Design review of the part shown in the three views and the two pictorial views. Dimensions are in mm from the part's minimum x, y and z. Give positions to 0.01 mm unless a question says otherwise; leave off trailing zeros. Write each loop counter-clockwise with the first axis right and the second up, starting at its lowest first coordinate (ties: lowest second). Pieces come first, ordered by that corner, then holes.
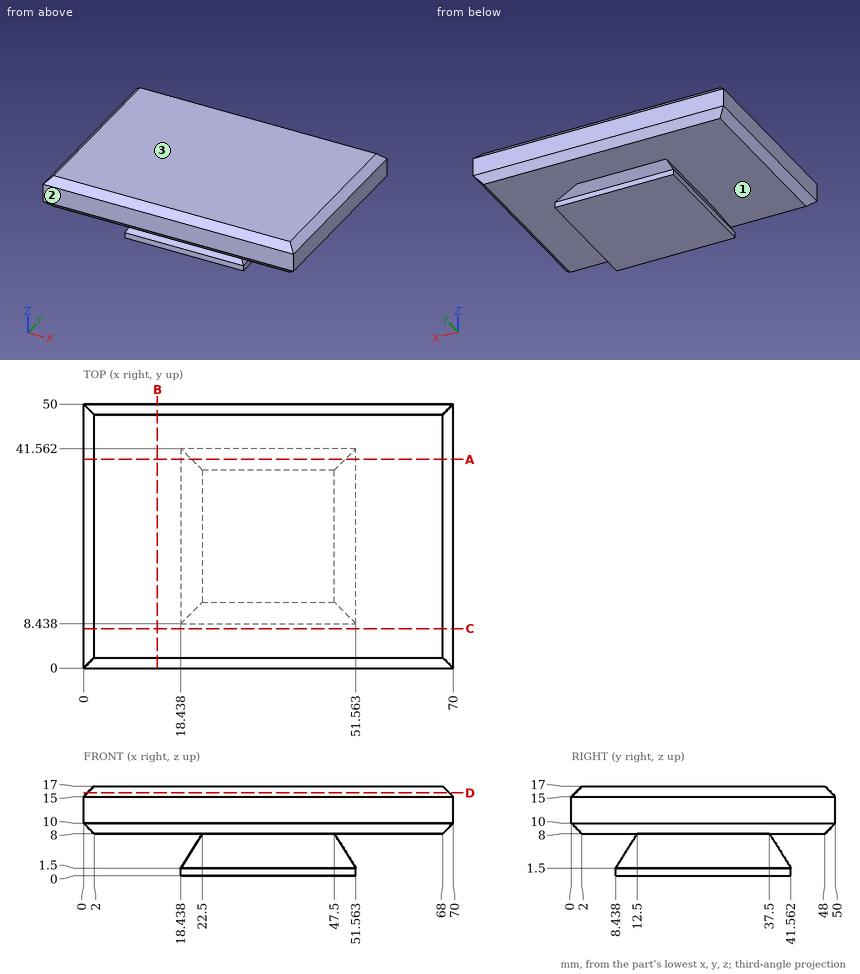
(1) Consider section D-D, the plane z = 15.75. Give the boundary of the cut face in (x, y).
Resolved:
outline: (0.75, 0.75) - (69.25, 0.75) - (69.25, 49.25) - (0.75, 49.25) - close
(2) Mouldability with a two-part tool opening along Z and no side actions: class the marked faces 1, 2 and 3 as pulls with the +Z half, pulls with the -Z half, needs draft (parallel to the pull), parting line crosses it, or undercut.
Resolved:
face 1: undercut
face 2: needs draft
face 3: pulls with the +Z half
(3) To check wall thickness, follow L1, parallel to Z at x = 17, y = 30.5; L2, parallel to Y at x = 50, z = 1; L3, parallel to X at y = 31, z = 1.75 (1 decimal). State the ranges of each line that lie inside material, in increasing order.
Resolved:
L1: z = 8 to 17
L2: y = 8.44 to 41.56
L3: x = 18.6 to 51.4
(4) Consider section A-A, the plane y = 39.5. Give the boundary of the cut face in (x, z).
Resolved:
outline: (0, 10) - (2, 8) - (68, 8) - (70, 10) - (70, 15) - (68, 17) - (2, 17) - (0, 15) - close; (18.44, 0) - (51.56, 0) - (51.56, 1.5) - (49.5, 4.8) - (20.5, 4.8) - (18.44, 1.5) - close
(5) Clearance check with flat-ended pins moving along their axes: P1, Ø0.8, axis at x = 31, z = 0.5, coming from the -Y side; P2, Ø1.5, axis at x = 63, y = 20.5, coming from the -Z side; P3, Ø1.5, axis at x = 58.5, z = 8.5, coming from the +Y side. State where each tip first meets the part, or that it passes through.
Resolved:
P1: stops at y = 8.44
P2: stops at z = 8
P3: stops at y = 49.25
(6) Consider section B-B, the plane x = 14. Give the boundary of the cut face in (y, z).
Resolved:
outline: (0, 10) - (2, 8) - (48, 8) - (50, 10) - (50, 15) - (48, 17) - (2, 17) - (0, 15) - close
(7) Consider section C-C, the plane y = 7.5. Give the boundary of the cut face in (x, z), then the cut area to 3 significant figures.
Resolved:
outline: (0, 10) - (2, 8) - (68, 8) - (70, 10) - (70, 15) - (68, 17) - (2, 17) - (0, 15) - close
area: 622 mm2
